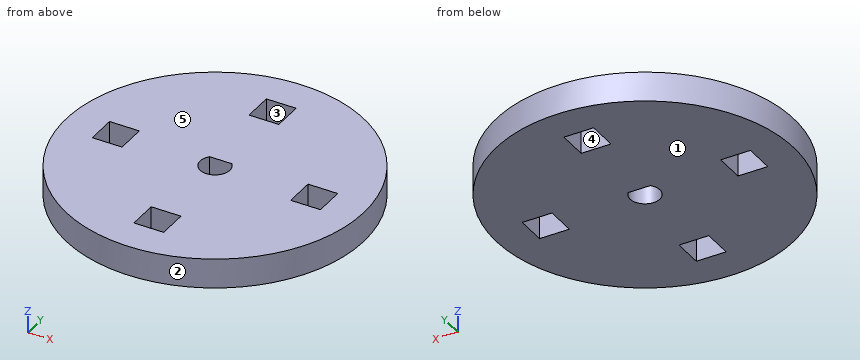
```python
from build123d import *

# Parameters (mm, degrees)
F1_R            = 15
F2_DEPTH        = 3
F3_W            = 3
F3_H            = 3
F4_DEPTH        = 3
F4_COPIES_COUNT = 4
F6_DEPTH        = 3


# Not quite as in the source:
# - a pattern or mirror of a feature is missing from the dataset's text; its kind, count and spacing are read off the source's solid


with BuildPart() as f2:
    # F1 (on Top) → F2 (new body)
    with BuildSketch(Plane.XY):
        Circle(F1_R)
    extrude(amount=-F2_DEPTH)

    # F3 (on face) → F4 (cut, through all)
    with BuildSketch(Plane.XY):
        with Locations((-10, 0)):
            Rectangle(F3_W, F3_H)
    f4 = extrude(amount=-F4_DEPTH, mode=Mode.SUBTRACT)

    # F4_copies: F4 ×4 about axis
    f4_copies_axis = Axis((0, 0, 0), (0, 0, 1))
    for i in range(1, F4_COPIES_COUNT):
        add(f4.rotate(f4_copies_axis, i * 360 / F4_COPIES_COUNT), mode=Mode.SUBTRACT)

    # F5 (on face) → F6 (cut, through all)
    with BuildSketch(Plane.XY):
        with BuildLine():
            Line((1.1180339887, 1), (-1.1180339887, 1))
            ThreePointArc((-1.1180339887, 1), (0, -1.5), (1.1180339887, 1))
        make_face()
    extrude(amount=-F6_DEPTH, mode=Mode.SUBTRACT)


solid = f2.part
```
Read the model definition and answer for the solid it produces. Units are mm, in the model's axes. Face numbers are marked on the shaded views. A direction names the side the tool comes from. Coordinates: 2 decimals unless noted, no trailing zeros. Loops run counter-clockwise (first coordinate to the right, second up) from the corner with the lowest first, then second, coordinate; pieces in that order, holes last. Notation, with made-up numbers: (19, 68) -> (35, 68) arc R31 cw to (35, 104) -> close; hole circle Ø4 at (82, -13.5). An arc over 180 degrees is marked (long way). Return JSON: item names as keys, results as strings.
Item 1: Find section D-D (y = 9.5). Determine the outline of the cut face in (x, z).
Answers:
{"outline": "(-11.61, -3) -> (-1.5, -3) -> (-1.5, 0) -> (-11.61, 0) -> close; (1.5, -3) -> (11.61, -3) -> (11.61, 0) -> (1.5, 0) -> close"}
Item 2: For the marked faces 4 and 5, determine the directions among +Z, -Z, +X, -X, +Y, -Y from which every point of the face is accessible in a straight line to the end or side of a thin tool.
Answers:
{"face 4": "+Z, -Z", "face 5": "+Z, +X, -X, +Y, -Y"}
Item 3: Find the intervals of material crossed by probe 1 along Y at (x, z) = (0.5, -1.8); probe 2 along Y at (x, z) = (10, -2.8); probe 3 along Y at (x, z) = (11, -2.35), in increasing order.
Answers:
{"probe 1": "y = -14.99 to -11.5, -8.5 to -1.41, 1 to 8.5, 11.5 to 14.99", "probe 2": "y = -11.18 to -1.5, 1.5 to 11.18", "probe 3": "y = -10.2 to -1.5, 1.5 to 10.2"}
Item 4: Find section B-B (x = 0). Determine the outline of the cut face in (y, z), plus the area to 3 significant figures.
Answers:
{"outline": "(-15, -3) -> (-11.5, -3) -> (-11.5, 0) -> (-15, 0) -> close; (-8.5, -3) -> (-1.5, -3) -> (-1.5, 0) -> (-8.5, 0) -> close; (1, -3) -> (8.5, -3) -> (8.5, 0) -> (1, 0) -> close; (11.5, -3) -> (15, -3) -> (15, 0) -> (11.5, 0) -> close", "area": "64.5 mm2"}
Item 5: For a pull along X with two mould halves and no side action, classify the marked faces 1, 2 and 3 as +X half, -X half, draft (parallel to the pull), parting line (faces both ways), or undercut.
Answers:
{"face 1": "draft", "face 2": "parting line", "face 3": "undercut"}
Item 6: Flat-ended cylindrical pins translate along their axes: P1, Ø1.5, axis at y = 9.5, z = -1.5, coming from the +X side; P2, Ø1.5, axis at y = 10, z = -1.5, coming from the +X side. Find the tip coordinate at first contact, or state that the pin passes through.
Answers:
{"P1": "stops at x = 12.18", "P2": "stops at x = 11.81"}
Item 7: Find section A-A (y = 0). Determine the outline of the cut face in (x, z), plus the area to 3 significant figures.
Answers:
{"outline": "(-15, -3) -> (-11.5, -3) -> (-11.5, 0) -> (-15, 0) -> close; (-8.5, -3) -> (-1.5, -3) -> (-1.5, 0) -> (-8.5, 0) -> close; (1.5, -3) -> (8.5, -3) -> (8.5, 0) -> (1.5, 0) -> close; (11.5, -3) -> (15, -3) -> (15, 0) -> (11.5, 0) -> close", "area": "63.0 mm2"}
Item 8: Find section C-C (z = -1). Determine the outline of the cut face in (x, y).
Answers:
{"outline": "circle Ø30 at (0, 0); hole (-11.5, -1.5) -> (-8.5, -1.5) -> (-8.5, 1.5) -> (-11.5, 1.5) -> close; hole (-1.5, -11.5) -> (1.5, -11.5) -> (1.5, -8.5) -> (-1.5, -8.5) -> close; hole (-1.5, 8.5) -> (1.5, 8.5) -> (1.5, 11.5) -> (-1.5, 11.5) -> close; hole (-1.12, 1) arc R1.5 ccw (long way) to (1.12, 1) -> close; hole (8.5, -1.5) -> (11.5, -1.5) -> (11.5, 1.5) -> (8.5, 1.5) -> close"}
